Solid Edge part; units mm, degrees
sketch "Sketch1" plane through (0, 0, 0) normal (0, 0, 1) x (1, 0, 0)
  line L0 (-3.5, -5.25) -> (3.5, -5.25)
  line L1 (3.5, -5.25) -> (3.5, 5.25)
  line L2 (3.5, 5.25) -> (-3.5, 5.25)
  line L3 (-3.5, 5.25) -> (-3.5, -5.25)
extrude "Protrusion1" add sketch "Sketch1" along normal mid plane 10
sketch "Sketch2" plane through (0, 5.25, 0) normal (0, 1, 0) x (0, 0, -1)
  circle A0 centre (0, 0) radius 2.5
extrude "ExtrudedCutout_3" cut sketch "Sketch2" against normal blind 9.5
sketch "Sketch3" plane through (0, -5.25, 0) normal (0, -1, 0) x (-1, 0, 0)
  line L0 (-3.5, 3.5) -> (3.5, 3.5)
  line L1 (3.5, 3.5) -> (3.5, 5)
  line L2 (3.5, 5) -> (-3.5, 5)
  line L3 (-3.5, 5) -> (-3.5, 3.5)
  line L4 (3.5, -3.5) -> (-3.5, -3.5)
  line L5 (-3.5, -3.5) -> (-3.5, -5)
  line L6 (-3.5, -5) -> (3.5, -5)
  line L7 (3.5, -5) -> (3.5, -3.5)
extrude "ExtrudedProtrusion_2" add sketch "Sketch3" along normal blind 7
sketch "Sketch4" plane through (0, -10.25, 3.5) normal (0, 0, -1) x (0, -1, 0)
  line L0 (0.75, -3.5) -> (2, -3.5)
  line L1 (2, -3.5) -> (2, 3.5)
  line L2 (2, 3.5) -> (0.75, 3.5)
  line L3 (0.75, 3.5) -> (0.75, -3.5)
extrude "Protrusion2" add sketch "Sketch4" along normal up to vertex (7 mm away)
fillet "Round_1" radius 0.75 16 edges at (3.5, -3.5, -5) (-3.5, -3.5, -5) (3.5, -12.25, 0) (-3.5, -12.25, 0) (0, -12.25, -5) (0, -12.25, 5) (-3.5, -3.5, 5) (0, -11, 3.5) (0, -11, -3.5) (0, -5.25, -3.5) (0, -5.25, 3.5) (3.5, -3.5, 5) (0, 5.25, 5) (-3.5, 5.25, 0) (3.5, 5.25, 0) (0, 5.25, -5)
properties material "ABS Plastic, medium impact"
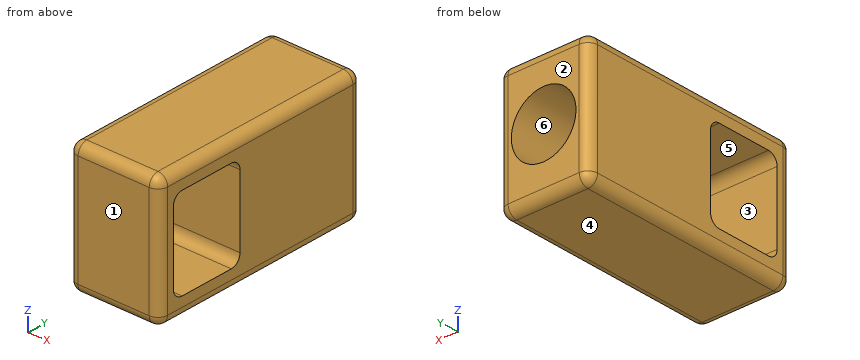
Design review of the part built by this model. Coordinates are the model's own, in mm. Face numbers are marked on the shaded views. A direction names the side the tool comes from. Give positions to 0.01 mm unless a question says otherwise; leave off trailing zeros. Order: outer loops, then holes, each group sorted by start corner. A loop starts at its lowest first (then second) coordinate and runs counter-clockwise, first axis right, second up.
1. For pin 1 Ø1.5 at (x, z) = (1, -1) entering from +Y; pin 2 Ø2 at (y, z) = (-6.5, 1.5) entering from -X, all flat-tipped, find the tip position at first contact; note any pin that passes through.
Solution:
pin 1: stops at y = -4.25
pin 2: passes through
2. Add section A-A, the plane z = 0. State the section outline as (x, y) points, then the cut area to 3 significant figures.
Solution:
outline: (-3.5, -11.5) arc R0.75 ccw to (-2.75, -12.25) - (2.75, -12.25) arc R0.75 ccw to (3.5, -11.5) - (3.5, -11) - (-3.5, -11) - close; (-3.5, -5.25) - (3.5, -5.25) - (3.5, 4.5) arc R0.75 ccw to (2.75, 5.25) - (2.5, 5.25) - (2.5, -4.25) - (-2.5, -4.25) - (-2.5, 5.25) - (-2.75, 5.25) arc R0.75 ccw to (-3.5, 4.5) - close
area: 34.3 mm2
3. To check wall thickness, follow L1, parallel to Y at x = 0.25, z = -1.5; L2, parallel to Y at x = 2.5, z = 0.75; L3, parallel to X at y = 3.25, z = 0. State the ranges of each line that lie inside material, in increasing order.
Solution:
L1: y = -12.25 to -11, -5.25 to -4.25
L2: y = -12.25 to -11, -5.25 to 5.25
L3: x = -3.5 to -2.5, 2.5 to 3.5
4. Add section C-C, the plane y = -8.5. State the section outline as (x, z) points.
Solution:
outline: (-3.5, -4.25) arc R0.75 ccw to (-2.75, -5) - (2.75, -5) arc R0.75 ccw to (3.5, -4.25) - (3.5, -3.5) - (-3.5, -3.5) - close; (-3.5, 3.5) - (3.5, 3.5) - (3.5, 4.25) arc R0.75 ccw to (2.75, 5) - (-2.75, 5) arc R0.75 ccw to (-3.5, 4.25) - close
5. Tool access review of the marked faces 4, 5 and 6: name each direction out of +Z, -Z, +X, -X, +Y, -Y from which nothing blocks a thin tool from reaching the whole face with its end or side.
Solution:
face 4: -Z, +X, -X, +Y, -Y
face 5: +X, -X
face 6: +Y
6. Add section D-D, the plane y = -3.5. State the section outline as (x, z) points, then the cut area to 3 significant figures.
Solution:
outline: (-3.5, -4.25) arc R0.75 ccw to (-2.75, -5) - (2.75, -5) arc R0.75 ccw to (3.5, -4.25) - (3.5, 4.25) arc R0.75 ccw to (2.75, 5) - (-2.75, 5) arc R0.75 ccw to (-3.5, 4.25) - close; hole circle Ø5 at (0, 0)
area: 49.9 mm2
7. Mouldability with a two-part tool opening along Y and no side actions: class the marked faces 1, 2 and 3 as +Y half, -Y half, draft (parallel to the pull), parting line (faces both ways), or undercut.
Solution:
face 1: -Y half
face 2: +Y half
face 3: undercut
8. Add section B-B, the plane x = -2. State the section outline as (y, z) points, then the cut area to 3 significant figures.
Solution:
outline: (-12.25, -4.25) arc R0.75 ccw to (-11.5, -5) - (4.5, -5) arc R0.75 ccw to (5.25, -4.25) - (5.25, -1.5) - (-4.25, -1.5) - (-4.25, 1.5) - (5.25, 1.5) - (5.25, 4.25) arc R0.75 ccw to (4.5, 5) - (-11.5, 5) arc R0.75 ccw to (-12.25, 4.25) - close; hole (-11, -2.75) arc R0.75 ccw to (-10.25, -3.5) - (-6, -3.5) arc R0.75 ccw to (-5.25, -2.75) - (-5.25, 2.75) arc R0.75 ccw to (-6, 3.5) - (-10.25, 3.5) arc R0.75 ccw to (-11, 2.75) - close
area: 106 mm2
